Read the model definition and answer for the solid it produces. Units are mm, in the model's axes. Face numbers are marked on the shaded views. A direction names the side the tool comes from. Round coordinates to 2 decimals unless told otherwise and drop trailing zeros. Order: outer loops, then holes, each group sorted by start corner. A loop starts at its lowest first (then second) coordinate and runs counter-clockwise, first axis right, second up. Notation, with made-up numbers: (39, 53.5) -> (74, 53.5) arc R25 cw to (74, 90.5) -> close; hole circle Ø7 at (20, 24). An arc over 180 degrees is marked (long way). Use a Markdown table: item, result. Add a question column.
1. Section C-C, the plane x = 0 is taken. Give the vertices of the cut face in (y, z) (3 decimals).
2. Given pin 1 (3 mm diameter, centred on x = -12.5, y = -32, fed in from -Z) (3 decimals); pin 2 (15 mm diameter, centred on x = 0, y = 0, fed in from +Z), each flat-ended and moving along its own axis, determine where each tip first touches the part or whether it passes through.
3. Consider L1, parallel to X at y = 3, z = 77; L2, parallel to Y at x = 0, z = 79.9. Determine where each line is inside the solid, lowest interval first. Write a range as [from, to].
4. Section D-D, the plane x = -33 is taken. Give the vertices of the cut face in (y, z) (3 decimals).
5. For the marked faces 4, 5 and 6, determine the directions among +Z, -Z, +X, -X, +Y, -Y from which every point of the face is accessible in a straight line to the end or side of a thin tool.
6. Section B-B, the plane z = 61.5 is taken. Give the vertices of the cut face in (x, y).
7. Section A-A, the plane y = 0 is taken. Give the vertices of the cut face in (x, z) (3 decimals), then the cut area to 3 significant figures.
8. The mould has two halves that part along Y. Classify the marked faces 1, 2 and 3: +Y half, -Y half, draft (parallel to the pull), parting line (faces both ways), or undercut.
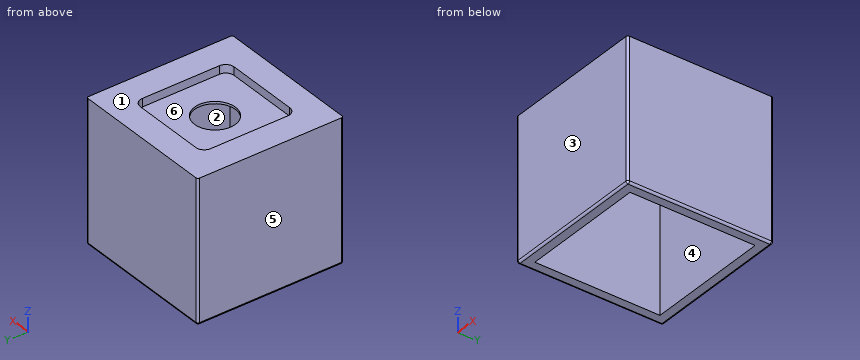
```python
from build123d import *

# Parameters (mm, degrees)
F0_W     = 88.9
F0_H     = 88.9
F1_DEPTH = 85.725
F2_T     = -6.35
F3_W     = 54.725456
F3_H     = 57.15
F4_DEPTH = 5
F5_R     = 5.08
F6_R     = 1.27
F7_R     = 12.425883
F8_DEPTH = 25.4


with BuildPart() as f1:
    # F0 (on Top) → F1 (new body)
    with BuildSketch(Plane.XY):
        Rectangle(F0_W, F0_H)
    extrude(amount=F1_DEPTH)

    # F2
    f2_openings = [f1.faces().sort_by_distance(p)[0] for p in [
        (0, 0, 0),
    ]]
    offset(amount=F2_T, openings=f2_openings)

    # F3 (on face) → F4 (cut)
    with BuildSketch(Plane.XY.offset(85.725)):
        Rectangle(F3_W, F3_H)
    extrude(amount=-F4_DEPTH, mode=Mode.SUBTRACT)

    # F5
    f5_edges = [f1.edges().sort_by_distance(p)[0] for p in [
        (-27.362728, 28.575, 83.225),
        (-27.362728, -28.575, 83.225),
        (27.362728, -28.575, 83.225),
        (27.362728, 28.575, 83.225),
    ]]
    fillet(f5_edges, radius=F5_R)

    # F6
    f6_edges = [f1.edges().sort_by_distance(p)[0] for p in [
        (44.45, -44.45, 42.8625),
        (44.45, 44.45, 42.8625),
        (-44.45, -44.45, 42.8625),
        (-44.45, 44.45, 42.8625),
        (-44.45, 0, 0),
        (0, -44.45, 0),
        (0, 44.45, 0),
        (44.45, 0, 0),
    ]]
    fillet(f6_edges, radius=F6_R)

    # F7 (on face) → F8 (cut)
    with BuildSketch(Plane.XY.offset(80.725)):
        Circle(F7_R)
    extrude(amount=-F8_DEPTH, mode=Mode.SUBTRACT)


solid = f1.part
```
Verdict:
| question | item | result |
|---|---|---|
| 1 | outline | (-44.45, 1.27) arc R1.27 ccw to (-43.18, 0) -> (-38.1, 0) -> (-38.1, 79.375) -> (-12.426, 79.375) -> (-12.426, 80.725) -> (-28.575, 80.725) -> (-28.575, 85.725) -> (-44.45, 85.725) -> close; (12.426, 79.375) -> (38.1, 79.375) -> (38.1, 0) -> (43.18, 0) arc R1.27 ccw to (44.45, 1.27) -> (44.45, 85.725) -> (28.575, 85.725) -> (28.575, 80.725) -> (12.426, 80.725) -> close |
| 2 | pin 1 | stops at z = 79.375 |
| 2 | pin 2 | passes through |
| 3 | L1 | x = [-44.45, -38.1], [38.1, 44.45] |
| 3 | L2 | y = [-44.45, -12.43], [12.43, 44.45] |
| 4 | outline | (-44.45, 1.27) arc R1.27 ccw to (-43.18, 0) -> (-38.1, 0) -> (-38.1, 79.375) -> (38.1, 79.375) -> (38.1, 0) -> (43.18, 0) arc R1.27 ccw to (44.45, 1.27) -> (44.45, 85.725) -> (-44.45, 85.725) -> close |
| 5 | face 4 | -Z |
| 5 | face 5 | +Z, -Z, -X, +Y, -Y |
| 5 | face 6 | +Z |
| 6 | outline | (-44.45, -43.18) arc R1.27 ccw to (-43.18, -44.45) -> (43.18, -44.45) arc R1.27 ccw to (44.45, -43.18) -> (44.45, 43.18) arc R1.27 ccw to (43.18, 44.45) -> (-43.18, 44.45) arc R1.27 ccw to (-44.45, 43.18) -> close; hole (-38.1, -38.1) -> (38.1, -38.1) -> (38.1, 38.1) -> (-38.1, 38.1) -> close |
| 7 | outline | (-44.45, 1.27) arc R1.27 ccw to (-43.18, 0) -> (-38.1, 0) -> (-38.1, 79.375) -> (-12.426, 79.375) -> (-12.426, 80.725) -> (-27.363, 80.725) -> (-27.363, 85.725) -> (-44.45, 85.725) -> close; (12.426, 79.375) -> (38.1, 79.375) -> (38.1, 0) -> (43.18, 0) arc R1.27 ccw to (44.45, 1.27) -> (44.45, 85.725) -> (27.363, 85.725) -> (27.363, 80.725) -> (12.426, 80.725) -> close |
| 7 | area | 1,260 mm2 |
| 8 | face 1 | draft |
| 8 | face 2 | undercut |
| 8 | face 3 | -Y half |
